Read the model definition and answer for the solid it produces. Units are mm, in the model's axes. Face numbers are marked on the shaded views. Coordinates: 2 decimals unless noted, no trailing zeros. Loops run counter-clockwise (first coordinate to the right, second up) from the corner with the lowest first, then second, coordinate; pieces in that order, holes last.
Q1. Flat-ended cylindrical pins translate along their axes: P1, Ø12, axis at x = 35, z = -2111, coming from the -Y side; P2, Ø10.5, axis at x = 75, y = 343, coming from the +Z side. Find the tip coordinate at first contact, or state that the pin passes through.
Q2. Section B-B (x = -77) is taken. Give the vertices of the cut face in (y, z).
Q3. Straight lines are drawn through the part: line 1 (Z direction, x = 5.5, y = 320.5); line 2 (Y direction, x = 75, z = -2100.8); line 3 (Y direction, x = 36.5, z = -2105.5). For each, find the intervals that lie inside material, in ascending order.
Q4. Section D-D (x = 8.5) is taken. Give the vertices of the cut face in (y, z).
Q5. Section A-A (y = 322) is taken. Give the vertices of the cut face in (x, z).
Q6. Section C-C (y = 343) is taken. Give the vertices of the cut face in (x, z), then the cut area to 3 significant figures.
Q7. The mould has two halves that part along Z. Classify the marked faces 1, 2 and 3: pulls with the +Z half, pulls with the -Z half, needs draft (parallel to the pull), parting line crosses it, or undercut.
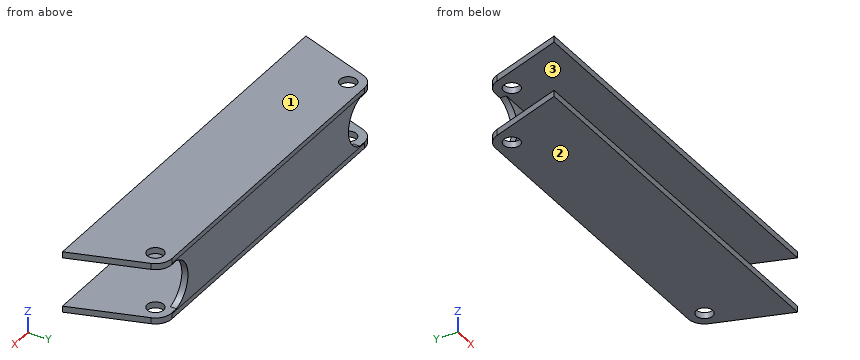
from build123d import *

# Parameters (mm, degrees)
BOSS_EXTRUDE5_START = 348
BOSS_EXTRUDE5_DEPTH = 3
BOSS_EXTRUDE6_START = -12
F_3DSKETCH1_R       = 4
BOSS_EXTRUDE6_DEPTH = 3


# Read off the part's stored shape, not the designer's step: Boss-Extrude5
with BuildPart() as part:
    # Boss-Extrude5 outline → Boss-Extrude5 (new body)
    with BuildSketch(Plane(origin=(0, 0, 0), x_dir=(1, 0, 0), z_dir=(0, 1, 0)).offset(BOSS_EXTRUDE5_START)):
        with BuildLine():
            ThreePointArc((-75, 2127.541936718), (-62.458063282, 2115), (-75, 2102.458063282))
            Line((-75, 2102.458063282), (75, 2102.458063282))
            ThreePointArc((75, 2102.458063282), (62.458063282, 2115), (75, 2127.541936718))
            Line((75, 2127.541936718), (-75, 2127.541936718))
        make_face()
    extrude(amount=BOSS_EXTRUDE5_DEPTH)

    # 3DSketch1 → Boss-Extrude6 (add)
    with BuildSketch(Plane(origin=(-82.570684984, 345.585484263, -2115), x_dir=(0.9804457750026082, -0.19678943640230048, 0), z_dir=(0, 0, -1)).offset(BOSS_EXTRUDE6_START)):
        with BuildLine():
            Line((0, 0), (-4.912403262, 37.281198271))
            Line((-4.912403262, 37.281198271), (180.830256509, 0))
            Line((180.830256509, 0), (161.912158463, -32.498077123))
            ThreePointArc((161.912158463, -32.498077123), (158.280606568, -35.768969819), (153.423992856, -36.31688537))
            Line((153.423992856, -36.31688537), (6.357126606, -6.798469909))
            ThreePointArc((6.357126606, -6.798469909), (2.088099295, -4.418908183), (0, 0))
        make_face()
        with Locations(Location((7.931442097, 1.045096291, 0), (0, 0, 348.650723519))):
            Circle(F_3DSKETCH1_R, mode=Mode.SUBTRACT)
        with Locations(Location((154.998308348, -28.47331917, 0), (0, 0, 348.650723519))):
            Circle(F_3DSKETCH1_R, mode=Mode.SUBTRACT)
    extrude(amount=-BOSS_EXTRUDE6_DEPTH)

    # Mirror4: part across plane


with BuildPart() as part_1:
    add(part.part)
    add(part.part.mirror(Plane.XY.offset(-2115)))


solid = part_1.part
Numbers:
1. P1: stops at y = 348
1. P2: stops at z = -2100
2. outline: (310, -2130) - (339.54, -2130) - (339.54, -2127) - (310, -2127) - close; (310, -2103) - (339.54, -2103) - (339.54, -2100) - (310, -2100) - close; (346.46, -2130) - (350.75, -2130) - (350.75, -2127) - (346.46, -2127) - close; (346.46, -2103) - (350.75, -2103) - (350.75, -2100) - (346.46, -2100) - close
3. line 1: z = -2130 to -2127, -2103 to -2100
3. line 2: y = 310 to 339, 347 to 351
3. line 3: y = 348 to 351
4. outline: (310, -2130) - (351, -2130) - (351, -2100) - (310, -2100) - (310, -2103) - (348, -2103) - (348, -2127) - (310, -2127) - close
5. outline: (-90.63, -2130) - (90.63, -2130) - (90.63, -2127) - (-90.63, -2127) - close; (-90.63, -2103) - (90.63, -2103) - (90.63, -2100) - (-90.63, -2100) - close
6. outline: (-83.45, -2130) - (-79, -2130) - (-79, -2127) - (-83.45, -2127) - close; (-83.45, -2103) - (-79, -2103) - (-79, -2100) - (-83.45, -2100) - close; (-71, -2130) - (71, -2130) - (71, -2127) - (-71, -2127) - close; (-71, -2103) - (71, -2103) - (71, -2100) - (-71, -2100) - close; (79, -2130) - (83.45, -2130) - (83.45, -2127) - (79, -2127) - close; (79, -2103) - (83.45, -2103) - (83.45, -2100) - (79, -2100) - close
6. area: 905 mm2
7. face 1: pulls with the +Z half
7. face 2: pulls with the -Z half
7. face 3: undercut
